Design review of the part shown in the three views and the two pictorial views. Dimensions are in mm from the part's minimum x, y and z. Round coordinates to 2 decimals unless told otherwise and drop trailing zeros. Order: outer loops, then holes, each group sorted by start corner. A loop starts at its lowest first (then second) coordinate and runs counter-clockwise, first axis right, second up.
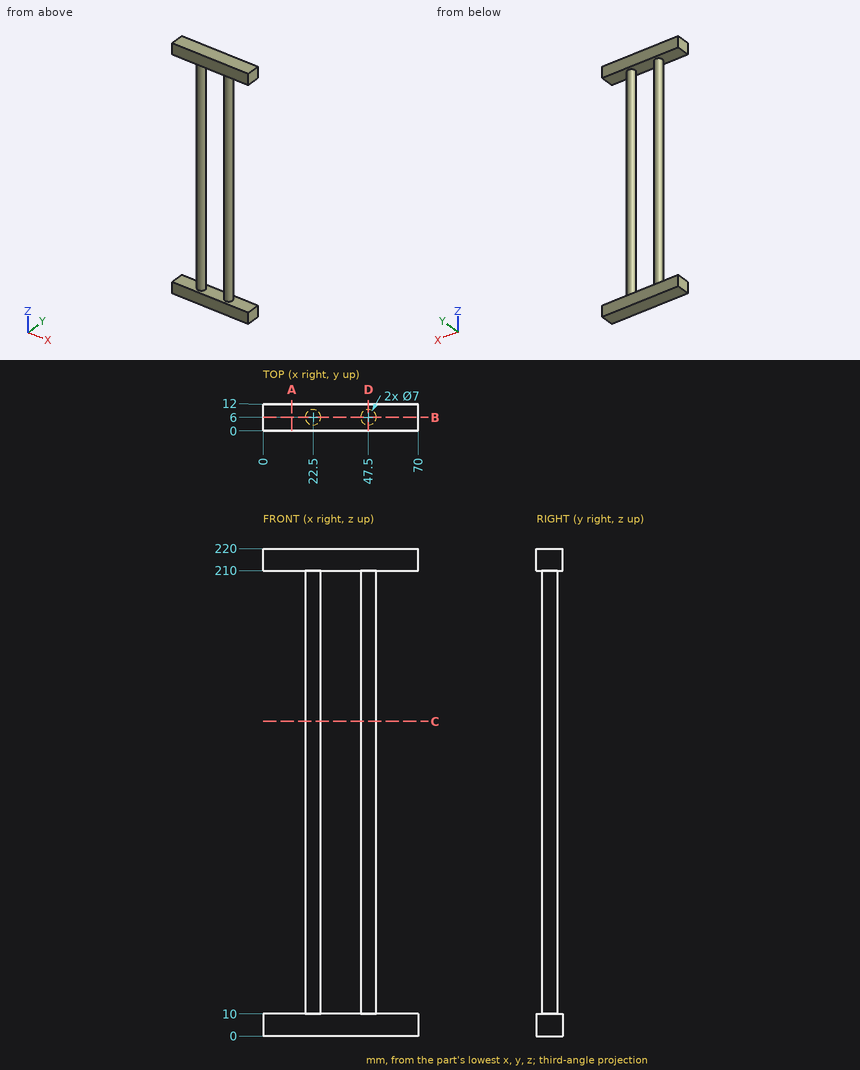
(1) Clearance check with flat-ended pins moving along their axes: P1, Ø8, axis at x = 49, z = 65, coming from the -Y side; P2, Ø5, axis at y = 4.5, z = 148, coming from the +X side; P3, Ø5, axis at x = 54.5, z = 163, coming from the +Y side. State where each tip first meets the part, or that it passes through.
(2) Wall thickness on L1, parallel to Z at x = 9.5, y = 3.5; L2, parallel to X at y = 7, z = 71.5; L3, parallel to X at y = 8.5, z = 69.5: over which ranges is each line inside the solid? List them lowest first.
(3) Add section D-D on x = 47.5. Give the boundary of the cut face in (y, z), plus the area to 3 significant figures.
(4) Add section B-B on y = 6. Give the boundary of the cut face in (x, z).
(5) Add section A-A on x = 13. Give the boundary of the cut face in (y, z).
(6) Add section C-C on z = 142. Give the boundary of the cut face in (x, y), plus the area to 3 significant figures.
Here are the results:
1. P1: stops at y = 2.5
1. P2: stops at x = 51
1. P3: passes through
2. L1: z = 0 to 10, 210 to 220
2. L2: x = 19.15 to 25.85, 44.15 to 50.85
2. L3: x = 20.05 to 24.95, 45.05 to 49.95
3. outline: (0, 0) - (12, 0) - (12, 10) - (9.5, 10) - (9.5, 210) - (12, 210) - (12, 220) - (0, 220) - (0, 210) - (2.5, 210) - (2.5, 10) - (0, 10) - close
3. area: 1,640 mm2
4. outline: (0, 0) - (70, 0) - (70, 10) - (51, 10) - (51, 210) - (70, 210) - (70, 220) - (0, 220) - (0, 210) - (19, 210) - (19, 10) - (0, 10) - close; hole (26, 10) - (44, 10) - (44, 210) - (26, 210) - close
5. outline: (0, 0) - (12, 0) - (12, 10) - (0, 10) - close; (0, 210) - (12, 210) - (12, 220) - (0, 220) - close
6. outline: circle Ø7 at (22.5, 6); circle Ø7 at (47.5, 6)
6. area: 77.0 mm2
